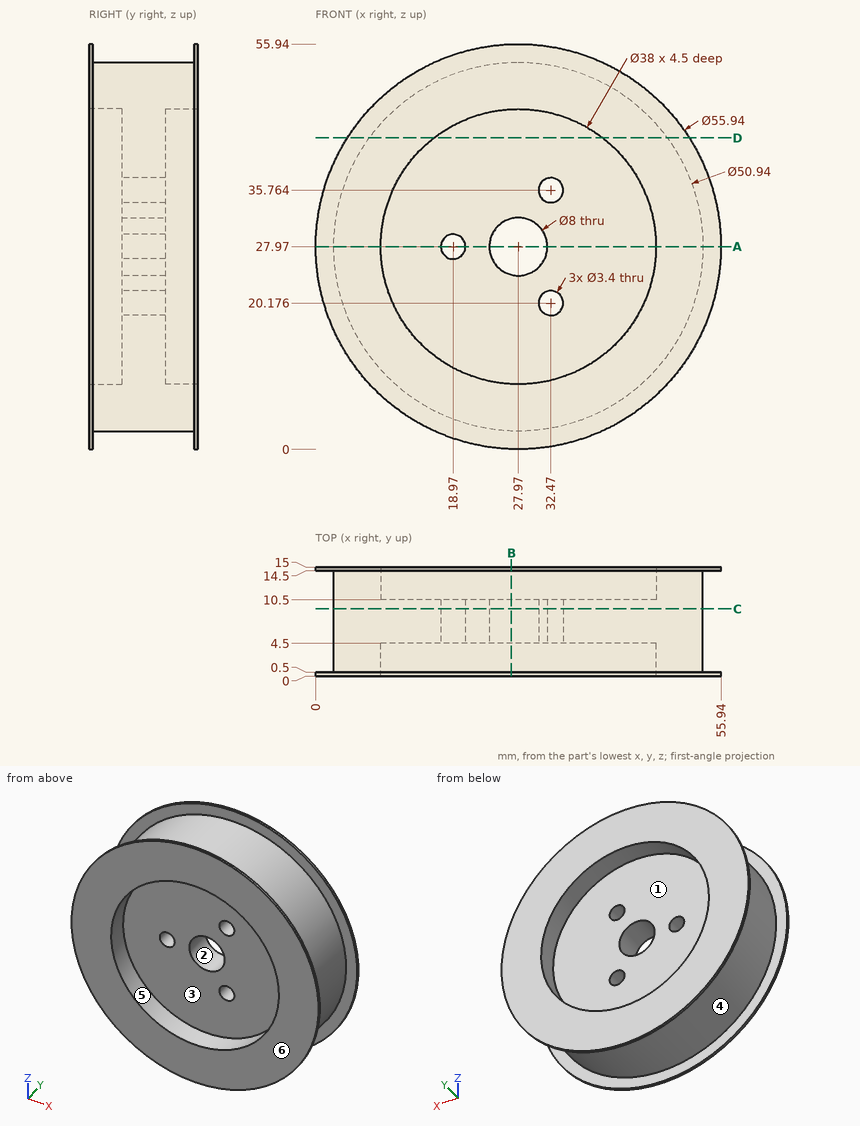
Verification items for this drawing (mm, ordinates from the low corner). A direction names the side the tool comes from. Give positions to 0.01 mm unless a question says otherwise; leave off trailing zeros. Write each loop counter-clockwise with the first axis right and the second up, starting at its lowest first coordinate (ties: lowest second). Pieces come first, ordered by that corner, then holes. Notation, with made-up numbers: (-17, 69.25) - (19, 69.25) arc R21 cw to (19, 86.25) - close; hole circle Ø7 at (-15, 86.25). An arc over 180 degrees is marked (long way). Answer as a JSON object with one key per item and string values. Group by question number.
1) Sectioned sample at D-D (z = 43). Record the cut outline in (x, y).
2) Sectioned sample at B-B (x = 27). Record the cut outline in (y, z) (1 decimal).
3) Depth check by flat-ended pin: P1, Ø1.5, axis at y = 8.5, z = 13.5, coming from the +X side; P2, Ø6, axis at y = 6.5, z = 13, coming from the -X side; P3, Ø4.5, axis at x = 32.47, z = 20.18, coming from the -Y side. Enter the tip coordinate at first touch or a pass-through.
4) Release check for a two-part mould opening along X. For the marked faces 3, 4, 5 and 6 record: pulls with the +X half, pulls with the -X half, needs draft (parallel to the pull), parting line crosses it, or undercut.
5) Sectioned sample at C-C (y = 9.25). Record the cut outline in (x, z), then the cut area to 3 significant figures.
6) Thickness scan on probe 1 along Y at (x, z) = (51, 12.5); probe 2 along Z at (x, y) = (27.5, 14.25); probe 3 along X at (y, z) = (12.05, 27.97). Record the ranges inside material, lowest first. Write a range as from..to.
7) Sectioned sample at A-A (z = 27.97). Record the cut outline in (x, y).
8) Access from +Z, -Z, +X, -X, +Y, -Y to the whole of each face (thin tool, end or side, straight path). Record for the marked faces 1 and 2.
Geometry results:
{
 "1": {"outline": "(4.38, 0) - (16.35, 0) - (16.35, 4.5) - (39.59, 4.5) - (39.59, 0) - (51.56, 0) - (51.56, 0.5) - (48.53, 0.5) - (48.53, 14.5) - (51.56, 14.5) - (51.56, 15) - (39.59, 15) - (39.59, 10.5) - (16.35, 10.5) - (16.35, 15) - (4.38, 15) - (4.38, 14.5) - (7.41, 14.5) - (7.41, 0.5) - (4.38, 0.5) - close"},
 "2": {"outline": "(0, 0) - (0.5, 0) - (0.5, 2.5) - (14.5, 2.5) - (14.5, 0) - (15, 0) - (15, 9) - (10.5, 9) - (10.5, 24.1) - (4.5, 24.1) - (4.5, 9) - (0, 9) - close; (0, 46.9) - (4.5, 46.9) - (4.5, 31.9) - (10.5, 31.9) - (10.5, 46.9) - (15, 46.9) - (15, 55.9) - (14.5, 55.9) - (14.5, 53.4) - (0.5, 53.4) - (0.5, 55.9) - (0, 55.9) - close"},
 "3": {"P1": "stops at x = 49.43", "P2": "stops at x = 5.49", "P3": "stops at y = 4.5"},
 "4": {"face 3": "undercut", "face 4": "parting line crosses it", "face 5": "undercut", "face 6": "needs draft"},
 "5": {"outline": "circle Ø50.94 at (27.97, 27.97); hole circle Ø3.4 at (18.97, 27.97); hole circle Ø8 at (27.97, 27.97); hole circle Ø3.4 at (32.47, 20.18); hole circle Ø3.4 at (32.47, 35.76)", "area": "1,960 mm^2"},
 "6": {"probe 1": "y = 0..0.5, 14.5..15", "probe 2": "z = 2.5..8.98, 46.96..53.44", "probe 3": "x = 2.5..8.97, 46.97..53.44"},
 "7": {"outline": "(0, 0) - (8.97, 0) - (8.97, 4.5) - (17.27, 4.5) - (17.27, 10.5) - (8.97, 10.5) - (8.97, 15) - (0, 15) - (0, 14.5) - (2.5, 14.5) - (2.5, 0.5) - (0, 0.5) - close; (20.67, 4.5) - (23.97, 4.5) - (23.97, 10.5) - (20.67, 10.5) - close; (31.97, 4.5) - (46.97, 4.5) - (46.97, 0) - (55.94, 0) - (55.94, 0.5) - (53.44, 0.5) - (53.44, 14.5) - (55.94, 14.5) - (55.94, 15) - (46.97, 15) - (46.97, 10.5) - (31.97, 10.5) - close"},
 "8": {"face 1": "+Y", "face 2": "+Y, -Y"}
}
